```python
from build123d import *

# Parameters (mm, degrees)
BOSS_EXTRUDE1_DEPTH   = 3
M4X0_7_TAPPED_HOLE1_D = 3.3
M6X1_0_TAPPED_HOLE2_D = 5


with BuildPart() as part:
    # Sketch1 → Boss-Extrude1 (new body)
    with BuildSketch(Plane(origin=(0, 0, 0), x_dir=(1, 0, 0), z_dir=(0, 1, 0))):
        Polygon((47, 40), (50, 37), (50, 3), (47, 0), (0, 0), (0, 40), align=None)
    extrude(amount=-BOSS_EXTRUDE1_DEPTH)

    # M4x0.7 Tapped Hole1 (through all)
    with Locations(Plane(origin=(0, 0, 0), x_dir=(1, 0, 0), z_dir=(0, 1, 0))):
        with Locations((45, 20)):
            Hole(M4X0_7_TAPPED_HOLE1_D / 2)

    # M6x1.0 Tapped Hole2 (through all)
    with Locations(Plane(origin=(0, 0, 0), x_dir=(1, 0, 0), z_dir=(0, 1, 0))):
        with Locations((8, 13.5), (8, 26.5)):
            Hole(M6X1_0_TAPPED_HOLE2_D / 2)


solid = part.part
```
Can you work these out from the model? Positions are in its coordinate system, mm. Round coordinates to 2 decimals unless told otherwise and drop trailing zeros. Loops run counter-clockwise (first coordinate to the right, second up) from the corner with the lowest first, then second, coordinate; pieces in that order, holes last.
Item 1: Suppose I cut it at B-B, the plane z = -13.5. Write out the boundary of the cut face in (x, y), then the cut area to 3 significant figures.
Item 2: If we mould it in two halves opening along Z, with no side actions, what happens to faces 1 (the cylindrical face through (8, -2, -29)), 2 (the flat face through (23, -1, -40)), 3 (the flat face through (49, -1, -2))? For each: +Z half, -Z half, draft (parallel to the pull), parting line (faces both ways), or undercut.
Item 3: Suppose I cut it at C-C, the plane x = 6.5. Write out the boundary of the cut face in (y, z), then the cut area to 3 significant figures.
Item 4: Suppose I cut it at A-A, the plane x = 45. Write out the boundary of the cut face in (y, z), then the cut area to 3 significant figures.
Item 5: Will this pin go through, and if not, where does the flat tip stop? pin 1 Ø3 at (x, z) = (45, -20) entering from +Y.
Item 6: Please list where these lines run through material, in increasing order: L1, parallel to Z at x = 8, y = -2.4; L2, parallel to X at y = -0.7, z = -26.5; L3, parallel to Z at x = 9, y = -2.6.
Item 7: Suppose I cut it at D-D, the plane y = -0.55. Write out the boundary of the cut face in (x, z).
Reported:
1. outline: (0, -3) - (5.5, -3) - (5.5, 0) - (0, 0) - close; (10.5, -3) - (50, -3) - (50, 0) - (10.5, 0) - close
1. area: 135 mm2
2. face 1: undercut
2. face 2: -Z half
2. face 3: +Z half
3. outline: (-3, -40) - (0, -40) - (0, -28.5) - (-3, -28.5) - close; (-3, -24.5) - (0, -24.5) - (0, -15.5) - (-3, -15.5) - close; (-3, -11.5) - (0, -11.5) - (0, 0) - (-3, 0) - close
3. area: 96.0 mm2
4. outline: (-3, -40) - (0, -40) - (0, -21.65) - (-3, -21.65) - close; (-3, -18.35) - (0, -18.35) - (0, 0) - (-3, 0) - close
4. area: 110 mm2
5. pin 1: passes through
6. L1: z = -40 to -29, -24 to -16, -11 to 0
6. L2: x = 0 to 5.5, 10.5 to 50
6. L3: z = -40 to -28.79, -24.21 to -15.79, -11.21 to 0
7. outline: (0, -40) - (47, -40) - (50, -37) - (50, -3) - (47, 0) - (0, 0) - close; hole circle Ø5 at (8, -26.5); hole circle Ø5 at (8, -13.5); hole circle Ø3.3 at (45, -20)
